Check sheet for the modelled part. Datum: model origin and axes. Units: mm. Round coordinates to 2 decimals unless told otherwise and drop trailing zeros. Order: outer loops, then holes, each group sorted by start corner. A loop starts at its lowest first (then second) coordinate and runs counter-clockwise, first axis right, second up.
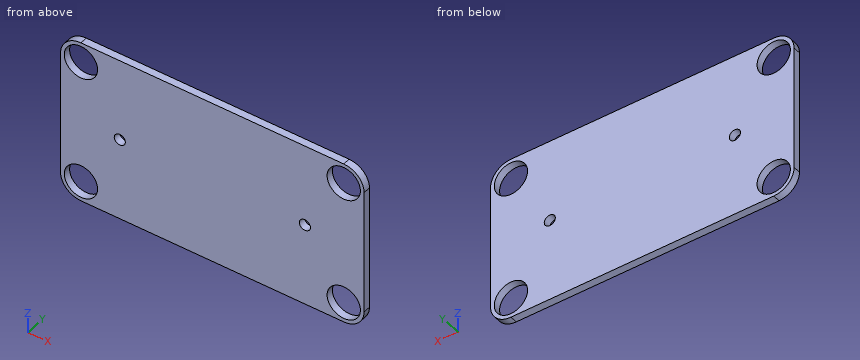
```python
from build123d import *

# Parameters (mm, degrees)
ESQUISSE1_W        = 82
ESQUISSE1_H        = 45
ESQUISSE1_R        = 4.5
ESQUISSE1_R_2      = 1.5
BOSS_EXTRU_1_DEPTH = 2
CONG_1_R           = 5.5


with BuildPart() as part:
    # Esquisse1 → Boss.-Extru.1 (new body)
    with BuildSketch(Plane(origin=(0, 0, 0), x_dir=(1, 0, 0), z_dir=(0, 1, 0))):
        Rectangle(ESQUISSE1_W, ESQUISSE1_H)
        with Locations((-35.5, 17)):
            Circle(ESQUISSE1_R, mode=Mode.SUBTRACT)
        with Locations((35.5, 17)):
            Circle(ESQUISSE1_R, mode=Mode.SUBTRACT)
        with Locations((35.5, -17)):
            Circle(ESQUISSE1_R, mode=Mode.SUBTRACT)
        with Locations((-35.5, -17)):
            Circle(ESQUISSE1_R, mode=Mode.SUBTRACT)
        with Locations((-25, 0)):
            Circle(ESQUISSE1_R_2, mode=Mode.SUBTRACT)
        with Locations((25, 0)):
            Circle(ESQUISSE1_R_2, mode=Mode.SUBTRACT)
    extrude(amount=BOSS_EXTRU_1_DEPTH)

    # Congé1
    cong_1_edges = [part.edges().sort_by_distance(p)[0] for p in [
        (-41, 1, -22.5),
        (41, 1, -22.5),
        (41, 1, 22.5),
        (-41, 1, 22.5),
    ]]
    fillet(cong_1_edges, radius=CONG_1_R)


solid = part.part
```
Item 1: Sectioned sample at A-A (x = -25). Record the cut outline in (y, z).
Answer:
outline: (0, -22.5) - (2, -22.5) - (2, -1.5) - (0, -1.5) - close; (0, 1.5) - (2, 1.5) - (2, 22.5) - (0, 22.5) - close
Item 2: Sectioned sample at B-B (z = 0). Record the cut outline in (x, y).
Answer:
outline: (-41, 0) - (-26.5, 0) - (-26.5, 2) - (-41, 2) - close; (-23.5, 0) - (23.5, 0) - (23.5, 2) - (-23.5, 2) - close; (26.5, 0) - (41, 0) - (41, 2) - (26.5, 2) - close
Item 3: Sectioned sample at C-C (y = 1.55). Record the cut outline in (x, z).
Answer:
outline: (-41, -17) arc R5.5 ccw to (-35.5, -22.5) - (35.5, -22.5) arc R5.5 ccw to (41, -17) - (41, 17) arc R5.5 ccw to (35.5, 22.5) - (-35.5, 22.5) arc R5.5 ccw to (-41, 17) - close; hole circle Ø9 at (-35.5, -17); hole circle Ø9 at (-35.5, 17); hole circle Ø3 at (-25, 0); hole circle Ø3 at (25, 0); hole circle Ø9 at (35.5, -17); hole circle Ø9 at (35.5, 17)
Item 4: Go/stop test with a flat-tipped pin: P1, Ø7, axis at x = 35.5, z = -17, coming from the +Y side. Record where the tip stops, or that it passes through.
Answer:
P1: passes through
Item 5: Scan lines: line 1 along Z through (x, y) = (35.5, 0.95); line 2 along X through (y, z) = (0.7, -17); line 3 along X through (y, z) = (0.5, 0). Record each from-to range of solid material in increasing order.
Answer:
line 1: z = -22.5 to -21.5, -12.5 to 12.5, 21.5 to 22.5
line 2: x = -41 to -40, -31 to 31, 40 to 41
line 3: x = -41 to -26.5, -23.5 to 23.5, 26.5 to 41
